Check sheet for the modelled part. Datum: model origin and axes. Units: mm. A direction names the side the tool comes from. Coordinates: 2 decimals unless noted, no trailing zeros. Write each loop counter-clockwise with the first axis right and the second up, starting at its lowest first coordinate (ties: lowest second). Pieces come first, ordered by that corner, then holes. Notation, with made-up numbers: (82.25, 16) -> (130.25, 16) arc R38 cw to (130.25, 55) -> close; hole circle Ø6 at (81.5, 5). An arc over 180 degrees is marked (long way). Put each result on its own line as item: value.
```python
from build123d import *

# Parameters (mm, degrees)
SKETCH1_W           = 40
SKETCH1_H           = 30
BOSS_EXTRUDE1_DEPTH = 4
SKETCH2_R           = 2.5
CUT_EXTRUDE1_DEPTH  = 26.317977802
SKETCH3_R           = 5
CUT_EXTRUDE2_DEPTH  = 2
BOSS_EXTRUDE2_DEPTH = 30


with BuildPart() as part:
    # Sketch1 → Boss-Extrude1 (new body)
    with BuildSketch(Plane(origin=(0, 0, 0), x_dir=(1, 0, 0), z_dir=(0, 1, 0))):
        Rectangle(SKETCH1_W, SKETCH1_H)
    extrude(amount=BOSS_EXTRUDE1_DEPTH)

    # Sketch2 → Cut-Extrude1 (cut, through all)
    with BuildSketch(Plane(origin=(0, 4, 0), x_dir=(1, 0, 0), z_dir=(0, 1, 0))):
        with Locations(Location((0, 0, 0), (0, 0, 270))):
            Circle(SKETCH2_R)
    extrude(amount=-CUT_EXTRUDE1_DEPTH, mode=Mode.SUBTRACT)

    # Sketch3 → Cut-Extrude2 (cut)
    with BuildSketch(Plane(origin=(0, 4, 0), x_dir=(1, 0, 0), z_dir=(0, 1, 0))):
        with Locations(Location((0, 0, 0), (0, 0, 270))):
            Circle(SKETCH3_R)
    extrude(amount=-CUT_EXTRUDE2_DEPTH, mode=Mode.SUBTRACT)

    # Sketch4 → Boss-Extrude2 (add)
    with BuildSketch(Plane(origin=(0, 0, -15), x_dir=(-1, 0, 0), z_dir=(0, 0, -1))):
        Polygon((-24, 0), (-20, 0), (-20, 4), (-20, 25), (-24, 25), align=None)
        Polygon((-66, 25), (-24, 25), (-20, 25), (-20, 29), (-66, 29), align=None)
        Polygon((-66, 9), (-66, 25), (-66, 29), (-70, 29), (-70, 9), align=None)
    extrude(amount=-BOSS_EXTRUDE2_DEPTH)


solid = part.part
```
Q1. Cross-section at D-D (z = 9.75). Record the cut outline in (x, y).
Recorded:
outline: (-20, 0) -> (24, 0) -> (24, 25) -> (66, 25) -> (66, 9) -> (70, 9) -> (70, 29) -> (20, 29) -> (20, 4) -> (-20, 4) -> close
Q2. Mould release check, pull along X, two halves, no side actions. Record for faces 1 (the flat face through (-20, 2, 0)), 2 (the cylindrical face through (-4.88, 3.01, -1.08)), 3 (the flat face through (-5, 4, -4)): released by +X, released by -X, zero draft, split by the parting line, or undercut.
Recorded:
face 1: released by -X
face 2: undercut
face 3: zero draft
Q3. Cross-section at A-A (x = 0). Record the cut outline in (y, z), plus the area to 3 significant figures.
Recorded:
outline: (0, -15) -> (4, -15) -> (4, -5) -> (2, -5) -> (2, -2.5) -> (0, -2.5) -> close; (0, 2.5) -> (2, 2.5) -> (2, 5) -> (4, 5) -> (4, 15) -> (0, 15) -> close
area: 90.0 mm2
Q4. Depth check by flat-ended pin: P1, Ø1.2, axis at x = 69, z = 4.5, coming from the -Y side; P2, Ø5, axis at x = 1.5, z = 0, coming from the +Y side; P3, Ø4.5, axis at x = 0, z = 0, coming from the -Y side; P4, Ø5, axis at y = 18.5, z = -2, coming from the -X side. Enter the tip coordinate at first touch or a pass-through.
Recorded:
P1: stops at y = 9
P2: stops at y = 2
P3: passes through
P4: stops at x = 20
Q5. Cross-section at B-B (z = 0). Record the cut outline in (x, y), plus the area to 3 significant figures.
Recorded:
outline: (-20, 0) -> (-2.5, 0) -> (-2.5, 2) -> (-5, 2) -> (-5, 4) -> (-20, 4) -> close; (2.5, 0) -> (24, 0) -> (24, 25) -> (66, 25) -> (66, 9) -> (70, 9) -> (70, 29) -> (20, 29) -> (20, 4) -> (5, 4) -> (5, 2) -> (2.5, 2) -> close
area: 494 mm2
Q6. Tool access check on faces 4 (the flat face through (68, 9, 0)), 5 (the flat face through (24, 13, 0)), 6 (the flat face through (20, 16, 0)). Record the directions out of +Z, -Z, +X, -X, +Y, -Y that give a thin tool (end or side, any length) a straight path to the whole face; none if there is none.
Recorded:
face 4: +Z, -Z, +X, -Y
face 5: +Z, -Z, -Y
face 6: +Z, -Z, -X, +Y
Q7. Cross-section at C-C (y = 10.5). Record the cut outline in (x, z).
Recorded:
outline: (20, -15) -> (24, -15) -> (24, 15) -> (20, 15) -> close; (66, -15) -> (70, -15) -> (70, 15) -> (66, 15) -> close
Q8. Material ranges on line 1 along X through (y, z) = (13.5, 11.25); line 2 along X through (y, z) = (3.3, 0); line 3 along X through (y, z) = (27.75, 5), recorded low to high.
Recorded:
line 1: x = 20 to 24, 66 to 70
line 2: x = -20 to -5, 5 to 24
line 3: x = 20 to 70
